Part model, mm, in its own coordinate system. A direction names the side the tool comes from. Round coordinates to 2 decimals unless told otherwise and drop trailing zeros. Write each loop counter-clockwise with the first axis right and the second up, starting at its lowest first coordinate (ties: lowest second). Pieces come first, ordered by that corner, then holes.
```python
from build123d import *

# Parameters (mm, degrees)
F4_DEPTH  = 30.001
F5_W      = 6
F5_H      = 7
F6_DEPTH  = 13
F7_W      = 50.395424
F7_H      = 8.032865
F8_DEPTH  = 30.001
F9_W      = 10
F9_H      = 4
F10_DEPTH = 1


with BuildPart() as f1:
    # F0 (on Right) → F1 (revolve)
    with BuildSketch(Plane.YZ):
        with BuildLine():
            Line((-30, 0), (0, 0))
            ThreePointArc((0, 0), (-15, 15), (-30, 0))
        make_face()
    revolve(axis=Axis((0, -15, 0), (0, -1, 0)))

    # F3 (on offset) → F4 (cut, through all)
    with BuildSketch(Plane.XY.offset(15)):
        with BuildLine():
            Line((15, 0), (0, 0))
            Line((0, 0), (-15, 0))
            ThreePointArc((-15, 0), (0, -3), (15, 0))
        make_face()
    extrude(amount=-F4_DEPTH, mode=Mode.SUBTRACT)

    # F5 (on Front) → F6 (cut)
    with BuildSketch(Plane.XZ):
        Rectangle(F5_W, F5_H)
    extrude(amount=F6_DEPTH, mode=Mode.SUBTRACT)

    # F7 (on Front) → F8 (cut, through all)
    with BuildSketch(Plane.XZ):
        with Locations((-1.727619, 13.516432)):
            Rectangle(F7_W, F7_H)
    extrude(amount=F8_DEPTH, mode=Mode.SUBTRACT)

    # F9 (on face) → F10 (cut)
    with BuildSketch(Plane.XY.offset(9.5)):
        with Locations((0, -15)):
            Rectangle(F9_W, F9_H)
        Polygon((-5, -17), (-5, -13), (-5, -10), (-10, -15), (-5, -20), align=None)
        Polygon((5, -10), (5, -13), (5, -17), (5, -20), (10, -15), align=None)
    extrude(amount=-F10_DEPTH, mode=Mode.SUBTRACT)


solid = f1.part
```
Q1. Cut at B-B on x = 6.5. Write the cut outline in (y, z), plus the area to 3 significant figures.
Values follow:
outline: (-24.62, 9.5) arc R13.52 ccw (long way) to (-2.45, -5.04) - (-2.45, 5.04) arc R13.52 ccw to (-5.38, 9.5) - (-11.5, 9.5) - (-11.5, 8.5) - (-18.5, 8.5) - (-18.5, 9.5) - close
area: 507 mm2
Q2. Cut at A-A on y = -8.5. Write the cut outline in (x, z), plus the area to 3 significant figures.
Values follow:
outline: (-9.62, 9.5) arc R13.52 ccw (long way) to (9.62, 9.5) - close; hole (-3, -3.5) - (3, -3.5) - (3, 3.5) - (-3, 3.5) - close
area: 479 mm2
Q3. Cut at D-D on z = -5.25. Write the cut outline in (x, y), plus the area to 3 significant figures.
Values follow:
outline: (-6.37, -2.48) arc R14.05 ccw (long way) to (6.37, -2.48) arc R39 cw to start
area: 603 mm2
Q4. Wall check: L1, parallel to Z at x = 1.75, y = -4.75; L2, parallel to X at y = -12.25, z = -1.25; L3, parallel to Z at x = -1.5, y = -9.5. Give the ranges that are in metal, low to high.
Values follow:
L1: z = -10.81 to -3.5, 3.5 to 9.5
L2: x = -14.69 to -3, 3 to 14.69
L3: z = -13.87 to -3.5, 3.5 to 9.5
Q5. Mould opens along Y. For faces 1 (the flat face through (-0.2, -17.4, 9.5)), 2 (the flat face through (-8, -17, 9)), 3 (the cylindrical face through (3.386, -2.853, 0.126)) say: +Y half, -Y half, draft (parallel to the pull), parting line (faces both ways), or undercut.
Values follow:
face 1: draft
face 2: undercut
face 3: +Y half
Q6. Drop flat-ended pins along their axis: pin 1 (6 mm diameter, centred on y = -22.5, z = -8.5, fed in from -X); pin 2 (1.5 mm diameter, centred on y = -17.5, z = -9.5, fed in from +X); pin 3 (4 mm diameter, centred on y = -15.5, z = -4, fed in from +X); pin 4 (8 mm diameter, centred on x = 4.5, y = -15, fed in from +Z). Give the stop position or say it passes through.
Values follow:
pin 1: stops at x = -12.47
pin 2: stops at x = 11.94
pin 3: stops at x = 14.86
pin 4: stops at z = 9.5
Q7. Which spindle directions (+Z, -Z, +X, -X, +Y, -Y) get a long thin tool onto all of the face, cutting with end or side? Do faces 4 (the flat face through (0, -8, -3.5)), 5 (the flat face through (5, -11, 9)). Say none if no direction does.
Values follow:
face 4: +Y
face 5: +Z
Q8. Cut at C-C on y = -15.5. Write the cut outline in (x, z).
Values follow:
outline: (-11.6, 9.5) arc R14.99 ccw (long way) to (11.6, 9.5) - (9.5, 9.5) - (9.5, 8.5) - (-9.5, 8.5) - (-9.5, 9.5) - close
